Here's how the part is built. I have some questions about the finished solid (model axes, mm). A direction names the side the tool comes from. Coordinates: 2 decimals unless noted, no trailing zeros. Order: outer loops, then holes, each group sorted by start corner. A loop starts at its lowest first (then second) coordinate and runs counter-clockwise, first axis right, second up.
```python
from build123d import *

# Parameters (mm, degrees)
SKETCH2_W           = 30.48
SKETCH2_H           = 20.32
BOSS_EXTRUDE1_DEPTH = 3.81
SKETCH3_R           = 10.16
SKETCH3_R_2         = 7.62
BOSS_EXTRUDE2_DEPTH = 5.08
SKETCH4_R           = 3.81
CUT_EXTRUDE1_DEPTH  = 20.007619525
BOSS_EXTRUDE3_DEPTH = 3.81
SKETCH11_R          = 3.81
CUT_EXTRUDE3_DEPTH  = 3.81
BOSS_EXTRUDE5_START = -3.81
SKETCH12_R          = 3.791845508
BOSS_EXTRUDE5_DEPTH = 3.81


with BuildPart() as part:
    # Sketch2 → Boss-Extrude1 (new body)
    with BuildSketch(Plane(origin=(0, 0, 0), x_dir=(1, 0, 0), z_dir=(0, 1, 0))):
        Rectangle(SKETCH2_W, SKETCH2_H)
    extrude(amount=BOSS_EXTRUDE1_DEPTH)

    # Sketch3 → Boss-Extrude2 (add)
    with BuildSketch(Plane(origin=(0, 3.81, 0), x_dir=(1, 0, 0), z_dir=(0, 1, 0))):
        with Locations(Location((0, 0, 0), (0, 0, 270))):
            Circle(SKETCH3_R)
        with Locations(Location((0, 0, 0), (0, 0, 270))):
            Circle(SKETCH3_R_2, mode=Mode.SUBTRACT)
    extrude(amount=BOSS_EXTRUDE2_DEPTH)

    # Sketch4 → Cut-Extrude1 (cut, through all)
    with BuildSketch(Plane(origin=(0, 3.81, 0), x_dir=(1, 0, 0), z_dir=(0, 1, 0))):
        with Locations(Location((0, 0, 0), (0, 0, 270))):
            Circle(SKETCH4_R)
    extrude(amount=-CUT_EXTRUDE1_DEPTH, mode=Mode.SUBTRACT)

    # Sketch6 → Boss-Extrude3 (add)
    with BuildSketch(Plane(origin=(15.24, 0, 0), x_dir=(0, 0, -1), z_dir=(1, 0, 0))):
        with BuildLine():
            Line((-10.16, 3.81), (-10.16, -10.054809762))
            ThreePointArc((-10.16, -10.054809762), (0, -20.214809762), (10.16, -10.054809762))
            Line((10.16, -10.054809762), (10.16, 3.81))
            Line((10.16, 3.81), (-10.16, 3.81))
        make_face()
    extrude(amount=-BOSS_EXTRUDE3_DEPTH)

    # Sketch11 → Cut-Extrude3 (cut)
    with BuildSketch(Plane(origin=(15.24, 0, 0), x_dir=(0, 0, -1), z_dir=(1, 0, 0))):
        with Locations((0, -10.16)):
            Circle(SKETCH11_R)
    extrude(amount=-CUT_EXTRUDE3_DEPTH, mode=Mode.SUBTRACT)

    # Sketch12 → Boss-Extrude5 (add)
    with BuildSketch(Plane.ZY.offset(15.24).offset(BOSS_EXTRUDE5_START)):
        with BuildLine():
            Line((-10.16, 3.81), (-10.16, -10.054809762))
            ThreePointArc((-10.16, -10.054809762), (0, -20.214809762), (10.16, -10.054809762))
            Line((10.16, -10.054809762), (10.16, 3.81))
            Line((10.16, 3.81), (-10.16, 3.81))
        make_face()
        with Locations((0, -10.054809762)):
            Circle(SKETCH12_R, mode=Mode.SUBTRACT)
    extrude(amount=BOSS_EXTRUDE5_DEPTH)


solid = part.part
```
Q1. For faces 1 (the flat face through (11.43, -5, 0)), 2 (the flat face through (11, 3.81, 0)), 3 (the flat face through (3, 3.81, 3)), 4 (the cylindrical face through (-13.308, -13.756, -0.822)), which set-ups out of +Z, -Z, +X, -X, +Y, -Y let a thin tool reach every point of the face, with its end or its side?
Q2. Will these pins go through, and if not, where does the flat tip stop? pin 1 (1 mm diameter, centred on x = 5.5, z = 5, fed in from +Y); pin 2 (4.5 mm diameter, centred on x = 0.5, z = 2, fed in from +Y); pin 3 (6 mm diameter, centred on x = -1, z = 1, fed in from -Y).
Q3. We'd pull the mould along Z, two halves only. Please class faces 5 (the cylindrical face through (13.362, -6.382, 0.496)), 6 (the cylindrical face through (7.555, 6.314, -0.992)), 7 (the cylindrical face through (10.074, 6.314, -1.323)), 8 (the flat face through (-15.24, -6, 0)): pulls with the +Z half, pulls with the -Z half, needs draft (parallel to the pull), parting line crosses it, or undercut.
Q4. If we section it at C-C on y = -11: Write out the boundary of the cut face in (x, z), then the cut area to 3 significant figures.
Q5. If we section it at D-D on x = 12.5: Write out the boundary of the cut face in (y, z), then the cut area to 3 significant figures.
Q6. If we section it at A-A on z = 0: Write out the boundary of the cut face in (x, y), then the cut area to 3 significant figures.
Q7. I need wall thicknesses on L1, parallel to X at y = -10.75, z = -4; L2, parallel to Y at x = -13.1, z = 0; L3, parallel to Y at x = -8.5, z = 5. Which ranges of each line are inside material? Lowest first, please.
Reply:
1. face 1: +Z, -Z, -Y
1. face 2: +X, +Y
1. face 3: +Y
1. face 4: -X
2. pin 1: stops at y = 8.89
2. pin 2: stops at y = 3.81
2. pin 3: stops at y = 0
3. face 5: undercut
3. face 6: undercut
3. face 7: parting line crosses it
3. face 8: needs draft
4. outline: (-15.24, -10.12) - (-11.43, -10.12) - (-11.43, -3.67) - (-15.24, -3.67) - close; (-15.24, 3.67) - (-11.43, 3.67) - (-11.43, 10.12) - (-15.24, 10.12) - close; (11.43, -10.12) - (15.24, -10.12) - (15.24, -3.72) - (11.43, -3.72) - close; (11.43, 3.72) - (15.24, 3.72) - (15.24, 10.12) - (11.43, 10.12) - close
4. area: 97.9 mm2
5. outline: (-10.05, -10.16) - (3.81, -10.16) - (3.81, 10.16) - (-10.05, 10.16) arc R10.16 ccw to start; hole circle Ø7.62 at (-10.16, 0)
5. area: 398 mm2
6. outline: (-15.24, -20.21) - (-11.43, -20.21) - (-11.43, -13.85) - (-15.24, -13.85) - close; (-15.24, -6.26) - (-11.43, -6.26) - (-11.43, 0) - (-3.81, 0) - (-3.81, 3.81) - (-7.62, 3.81) - (-7.62, 8.89) - (-10.16, 8.89) - (-10.16, 3.81) - (-15.24, 3.81) - close; (3.81, 0) - (11.43, 0) - (11.43, -6.35) - (15.24, -6.35) - (15.24, 3.81) - (10.16, 3.81) - (10.16, 8.89) - (7.62, 8.89) - (7.62, 3.81) - (3.81, 3.81) - close; (11.43, -20.21) - (15.24, -20.21) - (15.24, -13.97) - (11.43, -13.97) - close
6. area: 209 mm2
7. L1: x = -15.24 to -11.43, 11.43 to 15.24
7. L2: y = -20.21 to -13.85, -6.26 to 3.81
7. L3: y = 0 to 8.89
